```python
from build123d import *

# Parameters (mm, degrees)
F0_R     = 6.25
F0_W     = 4
F0_H     = 18
F1_DEPTH = 6
F3_W     = 2
F3_H     = 2
F2_W     = 2
F2_H     = 2
F4_DEPTH = 18
F5_R     = 6.25
F6_DEPTH = 25
F8_W     = 3
F8_H     = 12.5
F9_DEPTH = 18


with BuildPart() as f1:
    # F0 (on Front) → F1 (new body)
    with BuildSketch(Plane.XZ):
        Polygon((0, 18), (0, 0), (23, 0), (23, 18), (19, 18), (4, 18), align=None)
        with Locations((11.5, 9)):
            Circle(F0_R, mode=Mode.SUBTRACT)
        with Locations((2, 27)):
            Rectangle(F0_W, F0_H)
        with Locations((21, 27)):
            Rectangle(F0_W, F0_H)
    extrude(amount=F1_DEPTH)

    # F3 (on face) + F2 (on face) → F4 (cut)
    with BuildSketch(Plane.XY.offset(36)):
        with Locations((20, -3)):
            Rectangle(F3_W, F3_H)
    with BuildSketch(Plane.XY.offset(36)):
        with Locations((3, -3)):
            Rectangle(F2_W, F2_H)
    extrude(amount=-F4_DEPTH, mode=Mode.SUBTRACT)

    # F5 (on face) → F6 (join)
    with BuildSketch(Plane.XZ.offset(6)):
        Polygon((19, 18), (4, 18), (0, 18), (0, 0), (23, 0), (23, 18), align=None)
        with Locations((11.5, 9)):
            Circle(F5_R, mode=Mode.SUBTRACT)
    extrude(amount=F6_DEPTH)

    # F7: F1 across plane


with BuildPart() as f1_1:
    add(f1.part)
    add(f1.part.mirror(Plane.YZ))

    # F8 (on face) → F9 (join)
    with BuildSketch(Plane.XY.offset(18)):
        with Locations((-13.5, -24.75)):
            Rectangle(F8_W, F8_H)
        with Locations((-9.5, -24.75)):
            Rectangle(F8_W, F8_H)
    extrude(amount=F9_DEPTH)


solid = f1_1.part
```
Check sheet for the modelled part. Datum: model origin and axes. Units: mm. A direction names the side the tool comes from. Round coordinates to 2 decimals unless told otherwise and drop trailing zeros. Loops run counter-clockwise (first coordinate to the right, second up) from the corner with the lowest first, then second, coordinate; pieces in that order, holes last. Notation, with made-up numbers: (89, 51.25) -> (124, 51.25) arc R30 ccw to (124, 85.25) -> close; hole circle Ø3 at (60.5, 83.25). An arc over 180 degrees is marked (long way). Write item = value, one per line. Start each with the question number.
1) Sectioned sample at D-D, the plane z = 14. Record the cut outline in (x, y), plus the area to 3 significant figures.
2) Sectioned sample at B-B, the plane x = 11.5. Record the cut outline in (y, z).
3) Gauge pin test, flat ends, axial feed: pin 1 Ø2 at (x, z) = (-3.5, 27.5) entering from -Y; pin 2 Ø6 at (y, z) = (-26.5, 28.5) entering from +X; pin 3 Ø1 at (x, y) = (12, -22) entering from +Z. Record the tip position at first contact, or that the pin passes through.
4) Set-up check for faces 1 (the flat face through (-10, -18.5, 27)), 2 (the flat face through (-20, -2, 27)), 3 (the flat face through (-11, -25, 27)), 4 (the flat face through (-15, -25, 27)): record each of +Z, -Z, +X, -X, +Y, -Y from which the full face is reachable in a straight line by a thin tool's end or side.
5) Sectioned sample at A-A, the plane z = 9. Record the cut outline in (x, y), plus the area to 3 significant figures.
6) Release check for a two-part mould opening along Z. For faces 5 (the flat face through (0, -15, 0)), 6 (the flat face through (-21, -3, 27)), 7 (the cylindrical face through (6.54, -15.28, 5.2)), 8 (the flat face through (-14, -25, 36)) record: released by +Z, released by -Z, zero draft, split by the parting line, or undercut.
7) Thickness scan on probe 1 along Z at (x, y) = (-11.5, -24); probe 2 along X at (y, z) = (-11, 8.5); probe 3 along X at (y, z) = (-3, 21). Record the ranges inside material, lowest first.
8) Sectioned sample at C-C, the plane y = -29. Record the cut outline in (x, z), plus the area to 3 significant figures.
Results are:
q1.outline = (-23, -31) -> (-15.25, -31) -> (-15.25, 0) -> (-23, 0) -> close; (-7.75, -31) -> (7.75, -31) -> (7.75, 0) -> (-7.75, 0) -> close; (15.25, -31) -> (23, -31) -> (23, 0) -> (15.25, 0) -> close
q1.area = 961 mm^2
q2.outline = (-31, 0) -> (0, 0) -> (0, 2.75) -> (-31, 2.75) -> close; (-31, 15.25) -> (0, 15.25) -> (0, 18) -> (-31, 18) -> close
q3.pin_1 = -6
q3.pin_2 = -8
q3.pin_3 = 18
q4.face_1 = +Z, +X, -X, +Y
q4.face_2 = +Z
q4.face_3 = +Z, +Y, -Y
q4.face_4 = +Z, -X, +Y, -Y
q5.outline = (-23, -31) -> (-17.75, -31) -> (-17.75, 0) -> (-23, 0) -> close; (-5.25, -31) -> (5.25, -31) -> (5.25, 0) -> (-5.25, 0) -> close; (17.75, -31) -> (23, -31) -> (23, 0) -> (17.75, 0) -> close
q5.area = 651 mm^2
q6.face_5 = released by -Z
q6.face_6 = zero draft
q6.face_7 = undercut
q6.face_8 = released by +Z
q7.probe_1 = 0 to 2.75, 15.25 to 18
q7.probe_2 = -23 to -17.73, -5.27 to 5.27, 17.73 to 23
q7.probe_3 = -23 to -21, -2 to 2, 21 to 23
q8.outline = (-23, 0) -> (23, 0) -> (23, 18) -> (-8, 18) -> (-8, 36) -> (-11, 36) -> (-11, 18) -> (-12, 18) -> (-12, 36) -> (-15, 36) -> (-15, 18) -> (-23, 18) -> close; hole circle Ø12.5 at (-11.5, 9); hole circle Ø12.5 at (11.5, 9)
q8.area = 691 mm^2
